from build123d import *

# Parameters (mm, degrees)
MEASURED_BUTTON_PCB_DEPTH         = 1.6
SKETCH_2_R                        = 1.5
MEASURED_BUTTON_MOUNT_HOLES_DEPTH = 2


with BuildPart() as part:
    # 草图1 → Measured_button_PCB (new body)
    with BuildSketch(Plane.XY):
        with BuildLine():
            Line((0.5, 0), (23.55, 0))
            ThreePointArc((23.55, 0), (23.903553391, 0.146446609), (24.05, 0.5))
            Line((24.05, 0.5), (24.05, 35.23))
            ThreePointArc((24.05, 35.23), (23.903553391, 35.583553391), (23.55, 35.73))
            Line((23.55, 35.73), (0.5, 35.73))
            ThreePointArc((0.5, 35.73), (0.146446609, 35.583553391), (0, 35.23))
            Line((0, 35.23), (0, 0.5))
            ThreePointArc((0, 0.5), (0.146446609, 0.146446609), (0.5, 0))
        make_face()
    extrude(amount=MEASURED_BUTTON_PCB_DEPTH)

    # 草图2 → Measured_button_mount_holes (cut)
    with BuildSketch(Plane.XY):
        with Locations((3.5, 3.36)):
            Circle(SKETCH_2_R)
        with Locations((20.55, 3.36)):
            Circle(SKETCH_2_R)
    extrude(amount=MEASURED_BUTTON_MOUNT_HOLES_DEPTH, mode=Mode.SUBTRACT)


solid = part.part
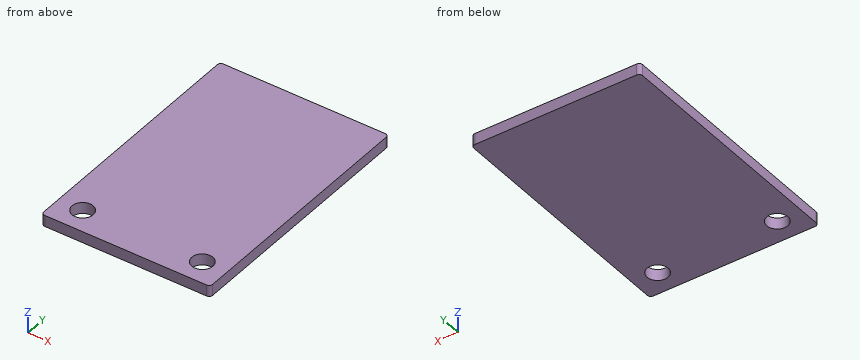
Geometry: final body of the model. Coordinates: model frame, mm. Coordinates: 2 decimals unless noted, no trailing zeros. Write each loop counter-clockwise with the first axis right and the second up, starting at its lowest first coordinate (ties: lowest second). Pieces come first, ordered by that corner, then holes. Notation, with made-up numbers: (5.25, -39) - (27.25, -39) arc R25 cw to (27.25, -22) - close; hole circle Ø2 at (-16.5, -26.75). An arc over 180 degrees is marked (long way). Return JSON: item names as keys, results as strings.
Item 1: Section query D-D (x = 19.5). Output: boundary loops of the cut face in (y, z), and give its area (3 significant figures).
Completed:
{"outline": "(0, 0) - (2.29, 0) - (2.29, 1.6) - (0, 1.6) - close; (4.43, 0) - (35.73, 0) - (35.73, 1.6) - (4.43, 1.6) - close", "area": "53.7 mm2"}
Item 2: Line query: L1, parallel to X at y = 3.36, z = 0.6; L2, parallel to X at y = 4.5, z = 0.2; L3, parallel to Y at x = 20.55, z = 1.1. Output: solid intervals per line, ascending.
Completed:
{"L1": "x = 0 to 2, 5 to 19.05, 22.05 to 24.05", "L2": "x = 0 to 2.53, 4.47 to 19.58, 21.52 to 24.05", "L3": "y = 0 to 1.86, 4.86 to 35.73"}
Item 3: Section query B-B (x = 3.5). Output: boundary loops of the cut face in (y, z), and give its area (3 significant figures).
Completed:
{"outline": "(0, 0) - (1.86, 0) - (1.86, 1.6) - (0, 1.6) - close; (4.86, 0) - (35.73, 0) - (35.73, 1.6) - (4.86, 1.6) - close", "area": "52.4 mm2"}
Item 4: Section query A-A (y = 3.36). Output: boundary loops of the cut face in (x, z).
Completed:
{"outline": "(0, 0) - (2, 0) - (2, 1.6) - (0, 1.6) - close; (5, 0) - (19.05, 0) - (19.05, 1.6) - (5, 1.6) - close; (22.05, 0) - (24.05, 0) - (24.05, 1.6) - (22.05, 1.6) - close"}
Item 5: Section query C-C (z = 1.3). Output: boundary loops of the cut face in (x, y), and give its area (3 significant figures).
Completed:
{"outline": "(0, 0.5) arc R0.5 ccw to (0.5, 0) - (23.55, 0) arc R0.5 ccw to (24.05, 0.5) - (24.05, 35.23) arc R0.5 ccw to (23.55, 35.73) - (0.5, 35.73) arc R0.5 ccw to (0, 35.23) - close; hole circle Ø3 at (3.5, 3.36); hole circle Ø3 at (20.55, 3.36)", "area": "845 mm2"}
